from build123d import *

# Parameters (mm, degrees)
SKETCH_1_R          = 10.15
EXTRUDE_1_DEPTH     = 32
CUT_EXTRUDE_1_DEPTH = 33
SKETCH_4_W          = 0.4
SKETCH_4_H          = 2
EXTRUDE_2_DEPTH     = 3
SKETCH_6_R          = 1
CUT_EXTRUDE_2_DEPTH = 4
SKETCH_6_4_R        = 3.05
EXTRUDE_3_DEPTH     = 2
SKETCH_7_R          = 1
EXTRUDE_4_DEPTH     = 6.8


with BuildPart() as part:
    # 草图1 → 凸台-拉伸1 (new body)
    with BuildSketch(Plane.XY):
        Circle(SKETCH_1_R)
    extrude(amount=EXTRUDE_1_DEPTH)

    # 草图3 → 切除-拉伸1 (cut, through all)
    with BuildSketch(Plane.XY.offset(32)):
        with BuildLine():
            ThreePointArc((6.670832032, 7.65), (0, 10.15), (-6.670832032, 7.65))
            Line((-6.670832032, 7.65), (6.670832032, 7.65))
        make_face()
        with BuildLine():
            Line((6.670832032, -7.65), (-6.670832032, -7.65))
            ThreePointArc((-6.670832032, -7.65), (0, -10.15), (6.670832032, -7.65))
        make_face()
    extrude(amount=-CUT_EXTRUDE_1_DEPTH, mode=Mode.SUBTRACT)

    # 草图4 → 凸台-拉伸2 (add)
    with BuildSketch(Plane(origin=(0, 0, 0), x_dir=(-1, 0, 0), z_dir=(0, 0, -1))):
        with Locations((6.2, 0)):
            Rectangle(SKETCH_4_W, SKETCH_4_H)
        with Locations((-6.2, 0)):
            Rectangle(SKETCH_4_W, SKETCH_4_H)
    extrude(amount=EXTRUDE_2_DEPTH)

    # 草图6 → 切除-拉伸2 (cut)
    with BuildSketch(Plane.XY.offset(32)):
        with Locations((-6.25, 0)):
            Circle(SKETCH_6_R)
        with Locations((6.25, 0)):
            Circle(SKETCH_6_R)
    extrude(amount=-CUT_EXTRUDE_2_DEPTH, mode=Mode.SUBTRACT)

    # 草图6<4> → 凸台-拉伸3 (add)
    with BuildSketch(Plane.XY.offset(32)):
        Circle(SKETCH_6_4_R)
    extrude(amount=EXTRUDE_3_DEPTH)

    # 草图7 → 凸台-拉伸4 (add)
    with BuildSketch(Plane.XY.offset(34)):
        Circle(SKETCH_7_R)
    extrude(amount=EXTRUDE_4_DEPTH)


solid = part.part
The model under review builds one solid part; all positions refer to its coordinate system, in mm. A direction names the side the tool comes from. Give positions to 0.01 mm unless a question says otherwise; leave off trailing zeros. Order: outer loops, then holes, each group sorted by start corner. A loop starts at its lowest first (then second) coordinate and runs counter-clockwise, first axis right, second up. Notation, with made-up numbers: (38.5, -4.5) -> (87.5, -4.5) arc R27 cw to (87.5, 25.5) -> close; hole circle Ø11 at (-25, 13). An arc over 180 degrees is marked (long way). Write item = value, one per line. Start each with the question number.
(1) For L1, parallel to Y at x = -6.25, z = 30.3; L2, parallel to Z at x = -6.75, y = -1.5; L3, parallel to Z at x = -2, y = 1.75, list the stretches that pass through material, from the lowest coordinate up. Write a range as from..to.
(2) Take a section at A-A (x = 0). Write out the cut boundary in (y, z).
(3) Take a section at B-B (y = 0). Write out the cut boundary in (x, z).
(4) Take a section at C-C (z = 18.5). Write out the cut boundary in (x, y).
(5) Tool access review of faces 1 (the flat face through (-0.1, -3.3, 32)), 2 (the flat face through (6.4, 0, -1)), 3 (the flat face through (6, 0, -1)): name each direction out of +Z, -Z, +X, -X, +Y, -Y from which nothing blocks a thin tool from reaching the whole face with its end or side.
(6) For pin 1 Ø1 at (y, z) = (0, -2) entering from +X; pin 2 Ø1 at (y, z) = (-0.5, -2) entering from -X; pin 3 Ø4 at (x, y) = (7, 2.5) entering from +Z, all flat-tipped, find the tip position at first contact; note any pin that passes through.
(7) Draft analysis for pull direction Y (two halves, no side actions). For faces 4 (the cylindrical face through (-10.15, 0.12, 15.78)), 5 (the flat face through (0, 7.65, 16)), 6 (the flat face through (0, 0, 0)), 7 (the flat face through (-6, 0, 28)), state which applies: +Y half, -Y half, draft (parallel to the pull), parting line (faces both ways), or undercut.
(8) Take a section at D-D (x = 3.75). Write out the cut boundary in (y, z), plus the area to 3 significant figures.
Returned:
q1.L1 = -7.65..-1, 1..7.65
q1.L2 = 0..32
q1.L3 = 0..34
q2.outline = (-7.65, 0) -> (7.65, 0) -> (7.65, 32) -> (3.05, 32) -> (3.05, 34) -> (1, 34) -> (1, 40.8) -> (-1, 40.8) -> (-1, 34) -> (-3.05, 34) -> (-3.05, 32) -> (-7.65, 32) -> close
q3.outline = (-10.15, 0) -> (-6.4, 0) -> (-6.4, -3) -> (-6, -3) -> (-6, 0) -> (6, 0) -> (6, -3) -> (6.4, -3) -> (6.4, 0) -> (10.15, 0) -> (10.15, 32) -> (7.25, 32) -> (7.25, 28) -> (5.25, 28) -> (5.25, 32) -> (3.05, 32) -> (3.05, 34) -> (1, 34) -> (1, 40.8) -> (-1, 40.8) -> (-1, 34) -> (-3.05, 34) -> (-3.05, 32) -> (-5.25, 32) -> (-5.25, 28) -> (-7.25, 28) -> (-7.25, 32) -> (-10.15, 32) -> close
q4.outline = (-6.67, -7.65) -> (6.67, -7.65) arc R10.15 ccw to (6.67, 7.65) -> (-6.67, 7.65) arc R10.15 ccw to start
q5.face_1 = +Z
q5.face_2 = -Z, +X, +Y, -Y
q5.face_3 = -Z, +Y, -Y
q6.pin_1 = 6.4
q6.pin_2 = -6.4
q6.pin_3 = 32
q7.face_4 = parting line
q7.face_5 = +Y half
q7.face_6 = draft
q7.face_7 = undercut
q8.outline = (-7.65, 0) -> (7.65, 0) -> (7.65, 32) -> (-7.65, 32) -> close
q8.area = 490 mm²
